from build123d import *

# Parameters (mm, degrees)
SKETCH1_W           = 44.5
SKETCH1_H           = 44.5
BASE_EXTRUDE_DEPTH  = 9.5
BOSS_EXTRUDE1_START = -15.75
SKETCH2_W           = 32
SKETCH2_H           = 31.5
BOSS_EXTRUDE1_DEPTH = 31.5
FILLET1_R           = 3
SKETCH3_W           = 4
SKETCH3_H           = 0.8
BOSS_EXTRUDE2_DEPTH = 6.5
BOSS_EXTRUDE3_DEPTH = 0.8
SKETCH5_R           = 1
CUT_EXTRUDE1_DEPTH  = 48.591517101


with BuildPart() as part:
    # Sketch1 → Base-Extrude (new, symmetric)
    with BuildSketch(Plane.XY):
        Rectangle(SKETCH1_W, SKETCH1_H)
    extrude(amount=BASE_EXTRUDE_DEPTH, both=True)

    # Sketch2 → Boss-Extrude1 (add)
    with BuildSketch(Plane(origin=(0, 0, 0), x_dir=(0, 0, -1), z_dir=(1, 0, 0)).offset(BOSS_EXTRUDE1_START)):
        Rectangle(SKETCH2_W, SKETCH2_H)
    extrude(amount=BOSS_EXTRUDE1_DEPTH)

    # Fillet1
    fillet1_edges = [part.edges().sort_by_distance(p)[0] for p in [
        (15.75, 15.75, -12.75),
        (15.75, -15.75, -12.75),
        (-15.75, -15.75, -12.75),
        (-15.75, 15.75, -12.75),
        (15.75, 15.75, 12.75),
        (15.75, -15.75, 12.75),
        (-15.75, -15.75, 12.75),
        (-15.75, 15.75, 12.75),
        (-22.25, 22.25, 0),
        (22.25, 22.25, 0),
        (22.25, -22.25, 0),
        (-22.25, -22.25, 0),
    ]]
    fillet(fillet1_edges, radius=FILLET1_R)

    # Sketch3 → Boss-Extrude2 (add)
    with BuildSketch(Plane.XY.offset(16)):
        with Locations((-5.25, -12.35)):
            Rectangle(SKETCH3_W, SKETCH3_H)
        with Locations((5.25, -12.35)):
            Rectangle(SKETCH3_W, SKETCH3_H)
    extrude(amount=BOSS_EXTRUDE2_DEPTH)

    # Sketch4 → Boss-Extrude3 (add)
    with BuildSketch(Plane(origin=(0, -11.95, 0), x_dir=(-1, 0, 0), z_dir=(0, 1, 0))):
        with BuildLine():
            Line((-7.25, 22.5), (-3.25, 22.5))
            ThreePointArc((-3.25, 22.5), (-5.25, 24.5), (-7.25, 22.5))
        make_face()
        with BuildLine():
            Line((3.25, 22.5), (7.25, 22.5))
            ThreePointArc((7.25, 22.5), (5.25, 24.5), (3.25, 22.5))
        make_face()
    extrude(amount=-BOSS_EXTRUDE3_DEPTH)

    # Sketch5 → Cut-Extrude1 (cut, through all)
    with BuildSketch(Plane(origin=(0, -11.95, 0), x_dir=(-1, 0, 0), z_dir=(0, 1, 0))):
        with Locations(Location((5.25, 22.5, 0), (0, 0, 90))):
            Circle(SKETCH5_R)
        with Locations(Location((-5.25, 22.5, 0), (0, 0, 90))):
            Circle(SKETCH5_R)
    extrude(amount=-CUT_EXTRUDE1_DEPTH, mode=Mode.SUBTRACT)


solid = part.part
Input: part model. Units: mm. Frame: model coordinates. A direction names the side the tool comes from. Coordinates: 2 decimals unless noted, no trailing zeros. Write each loop counter-clockwise with the first axis right and the second up, starting at its lowest first coordinate (ties: lowest second). Pieces come first, ordered by that corner, then holes. Notation, with made-up numbers: M 68.5,-22.75 L 92.5,-22.75 A18 ccw 92.5,-9.75 Z; hole C 5,77 d3. An arc over 180 degrees is marked long. Answer as a JSON object with one key per item and string values. Group by question number.
(1) Section A-A on x = 5.25. Output: boundary loops of the cut face in (y, z), plus the area to 3 significant figures.
(2) Section B-B on y = -7. Output: boundary loops of the cut face in (x, z), plus the area to 4 significant figures.
(3) Contact query for flat-ended pins moving along their axis: P1, Ø0.9, axis at y = -12.5, z = 20, coming from the -X side; P2, Ø1.6, axis at x = 5.25, z = 22.5, coming from the +Y side; P3, Ø5, axis at x = 3.5, z = -14, coming from the -Y side; P4, Ø9.5, axis at x = 7, y = 6.5, coming from the +Z side. Output: stop coordinate, or through.
(4) Section C-C on z = -11. Output: boundary loops of the cut face in (x, y), plus the area to 3 significant figures.
(5) Ray query, line 1 along X through (y, z) = (-12.5, 22.5); line 2 along X through (y, z) = (-12, 22); line 3 along Z through (x, y) = (11.5, 19.5). Return the intervals inside material, ascending. Write a range as [from, to].
(6) Mould query, pull axis Z, two halves, no side actions, for faces 1 (the face through (-20, 0, -9.5)), 2 (the face through (6.24, -12.34, 22.37)), 3 (the face through (-20, 0, 9.5)), 4 (the face through (15.75, 0, -13)). Classes: pulls with the +Z half, pulls with the -Z half, needs draft (parallel to the pull), parting line crosses it, or undercut.
(7) Set-up query: faces 5 (the face through (0, -15.75, 13)), 6 (the face through (-15.75, 0, -13)), 7 (the face through (0, 15.75, -13)). Return all of +Z, -Z, +X, -X, +Y, -Y with unobstructed straight access to the full face (end or side cutting, diameter ignored); none if empty.
Result set:
{
 "1": {"outline": "M -22.25,-9.5 L -15.75,-9.5 L -15.75,-16 L 15.75,-16 L 15.75,-9.5 L 22.25,-9.5 L 22.25,9.5 L 15.75,9.5 L 15.75,16 L -11.95,16 L -11.95,21.5 L -12.75,21.5 L -12.75,16 L -15.75,16 L -15.75,9.5 L -22.25,9.5 Z; M -12.75,23.5 L -11.95,23.5 L -11.95,24.5 L -12.75,24.5 Z", "area": "1,260 mm2"},
 "2": {"outline": "M -22.25,-9.5 L -15.75,-9.5 L -15.75,-16 L 15.75,-16 L 15.75,-9.5 L 22.25,-9.5 L 22.25,9.5 L 15.75,9.5 L 15.75,16 L -15.75,16 L -15.75,9.5 L -22.25,9.5 Z", "area": "1,255 mm2"},
 "3": {"P1": "stops at x = -7.25", "P2": "passes through", "P3": "stops at y = -15.75", "P4": "stops at z = 16"},
 "4": {"outline": "M -15.75,-12.75 A3 ccw -12.75,-15.75 L 12.75,-15.75 A3 ccw 15.75,-12.75 L 15.75,12.75 A3 ccw 12.75,15.75 L -12.75,15.75 A3 ccw -15.75,12.75 Z", "area": "985 mm2"},
 "5": {"line 1": "x = [-7.25, -6.25], [-4.25, -3.25], [3.25, 4.25], [6.25, 7.25]", "line 2": "x = [-7.25, -6.12], [-4.38, -3.25], [3.25, 4.38], [6.12, 7.25]", "line 3": "z = [-9.5, 9.5]"},
 "6": {"face 1": "pulls with the -Z half", "face 2": "undercut", "face 3": "pulls with the +Z half", "face 4": "needs draft"},
 "7": {"face 5": "+Z, +X, -X, -Y", "face 6": "-Z, -X, +Y, -Y", "face 7": "-Z, +X, -X, +Y"}
}
